Geometry: see drawing. Coordinates: mm, zero at the bounding-box minimum. A direction names the side the tool comes from. Give positions to 0.01 mm unless a question says otherwise; leave off trailing zeros. Order: outer loops, then holes, each group sorted by start corner. A loop starts at its lowest first (then second) coordinate and runs counter-clockwise, first axis right, second up. Notation, with made-up numbers: (-20.5, -27.5) - (-13.5, -27.5) arc R9 cw to (-13.5, -20.5) - close; hole circle Ø1 at (31, 25). An arc over 180 degrees is marked (long way). One line per item, written item: value.
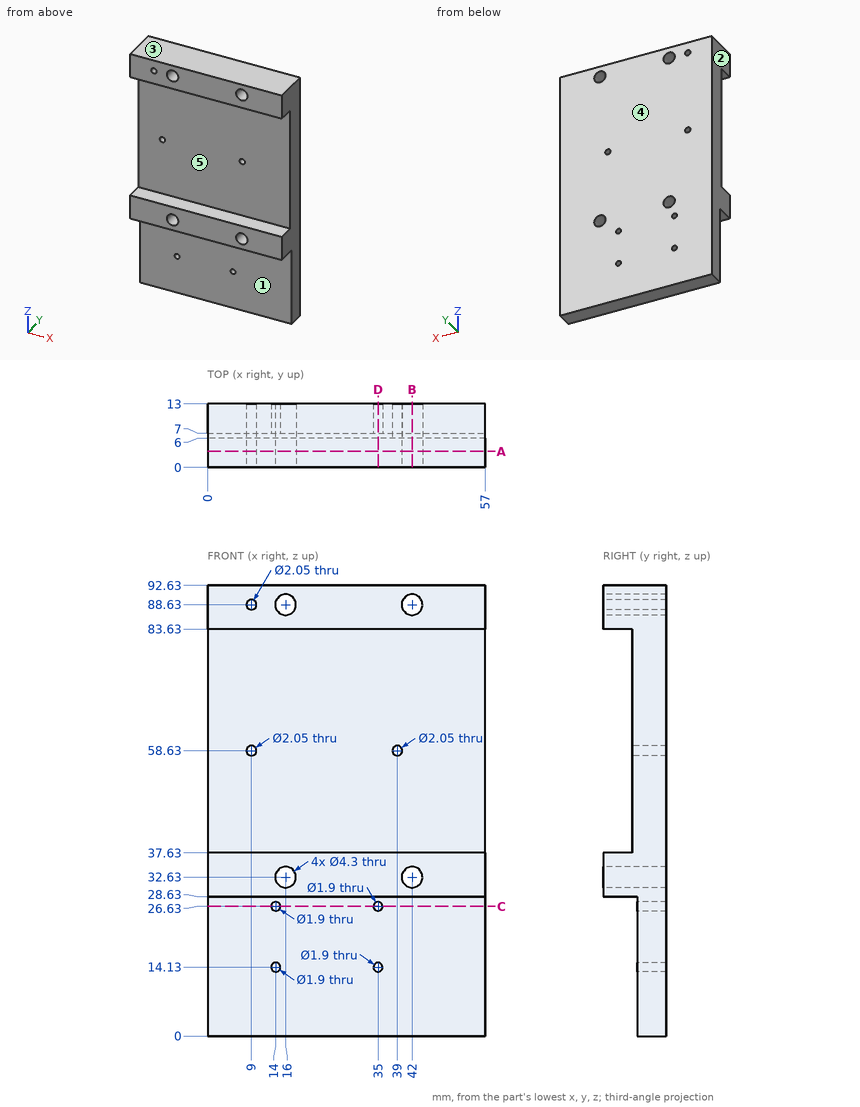
1) Material intervals for line 1 along Z through (x, y) = (42, 5.5); line 2 along X through (y, z) = (5.5, 32.63); line 3 along X through (y, z) = (4.25, 88.63) (3 decimals), sorted ascending.
Answers below:
line 1: 28.63 to 30.48, 34.78 to 37.63, 83.63 to 86.48, 90.78 to 92.63
line 2: 0 to 13.85, 18.15 to 39.85, 44.15 to 57
line 3: 0 to 7.975, 10.025 to 13.85, 18.15 to 39.85, 44.15 to 57
2) Section A-A, the plane y = 3.25. Return loops of the section in (x, z) (3 decimals), then the cut area to 3 significant figures.
Answers below:
outline: (0, 28.63) - (57, 28.63) - (57, 37.63) - (0, 37.63) - close; (0, 83.63) - (57, 83.63) - (57, 92.63) - (0, 92.63) - close; hole circle Ø2.05 at (9, 88.63); hole circle Ø4.3 at (16, 32.63); hole circle Ø4.3 at (16, 88.63); hole circle Ø4.3 at (42, 32.63); hole circle Ø4.3 at (42, 88.63)
area: 965 mm^2
3) Set-up query: the marked faces 1 and 2. Return all of +Z, -Z, +X, -X, +Y, -Y with unobstructed straight access to the full face (end or side cutting, diameter ignored); none if empty.
Answers below:
face 1: -Z, +X, -X, -Y
face 2: +Z, -Z, -X, +Y, -Y
4) First-contact query: pin 1 (1.5 mm diameter, centred on y = 8, z = 20.5, fed in from -X); pin 2 (2 mm diameter, centred on x = 7.5, y = 2, fed in from -Z); pin 3 (1 mm diameter, centred on x = 41.5, z = 22.5, fed in from -Y). Flat tips, straight axial feed; report the tip coordinate or a pass-through.
Answers below:
pin 1: x = 0
pin 2: z = 28.63
pin 3: y = 7
5) Mould query, pull axis Z, two halves, no side actions, for the marked faces 3, 4 and 5. Classes: released by +Z, released by -Z, zero draft, split by the parting line, or undercut.
Answers below:
face 3: released by +Z
face 4: zero draft
face 5: undercut
6) Section B-B, the plane x = 42. Return loops of the section in (y, z), then the cut area to 3 significant figures.
Answers below:
outline: (0, 28.63) - (7, 28.63) - (7, 0) - (13, 0) - (13, 30.48) - (0, 30.48) - close; (0, 34.78) - (13, 34.78) - (13, 86.48) - (0, 86.48) - (0, 83.63) - (6, 83.63) - (6, 37.63) - (0, 37.63) - close; (0, 90.78) - (13, 90.78) - (13, 92.63) - (0, 92.63) - close
area: 616 mm^2
7) Section D-D, the plane x = 35. Return loops of the section in (y, z), then the cut area to 3 significant figures.
Answers below:
outline: (0, 28.63) - (7, 28.63) - (7, 27.58) - (13, 27.58) - (13, 92.63) - (0, 92.63) - (0, 83.63) - (6, 83.63) - (6, 37.63) - (0, 37.63) - close; (7, 0) - (13, 0) - (13, 13.18) - (7, 13.18) - close; (7, 15.08) - (13, 15.08) - (13, 25.68) - (7, 25.68) - close
area: 705 mm^2
8) Section C-C, the plane z = 26.63. Return loops of the section in (x, y).
Answers below:
outline: (0, 7) - (13.05, 7) - (13.05, 13) - (0, 13) - close; (14.95, 7) - (34.05, 7) - (34.05, 13) - (14.95, 13) - close; (35.95, 7) - (57, 7) - (57, 13) - (35.95, 13) - close
